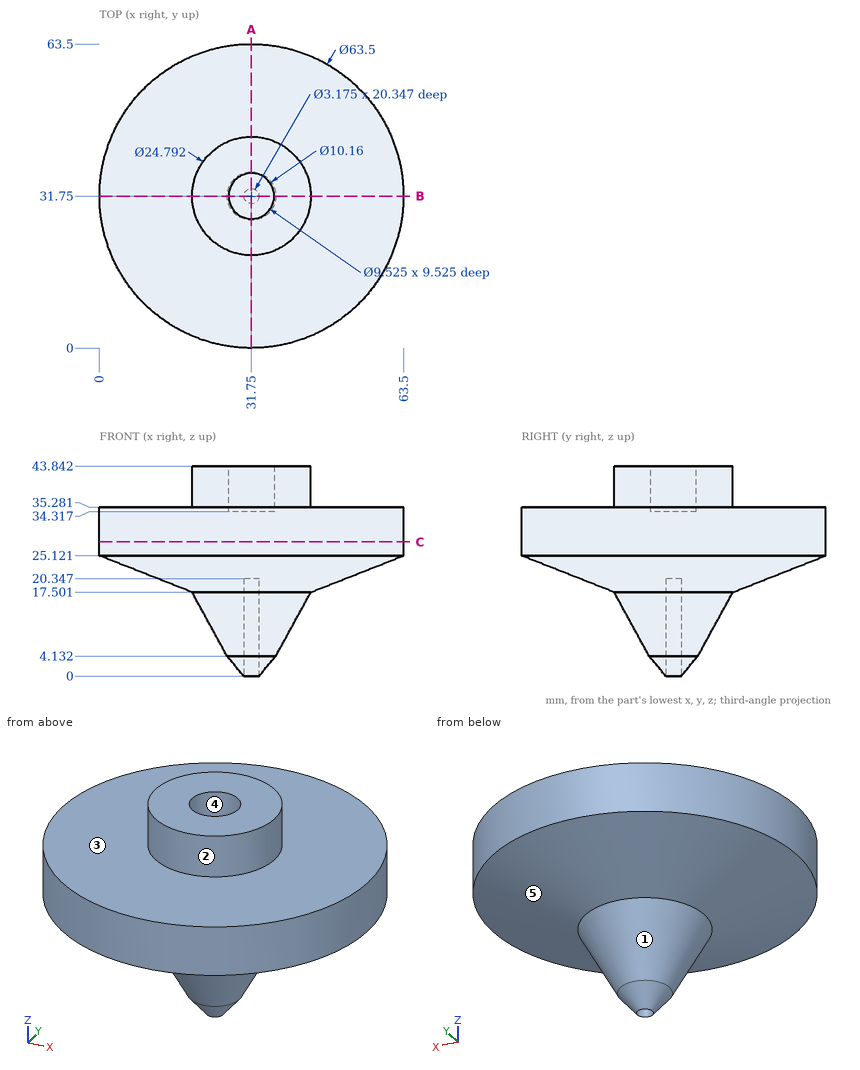
Check sheet for the drawn part. Datum: minimum x, y, z corner. Units: mm. A direction names the side the tool comes from. Round coordinates to 2 decimals unless told otherwise and drop trailing zeros. Write each loop counter-clockwise with the first axis right and the second up, starting at its lowest first coordinate (ties: lowest second). Pieces come first, ordered by that corner, then holes. Notation, with made-up numbers: (-15, 20) -> (21, 20) arc R26 cw to (21, 58) -> close; hole circle Ø3 at (-11.5, -16). An arc over 180 degrees is marked (long way). Put each result on its own line as item: value.
(1) Mould release check, pull along X, two halves, no side actions. Record for the marked faces 3, 4 and 5: released by +X, released by -X, zero draft, split by the parting line, or undercut.
Values found:
face 3: zero draft
face 4: undercut
face 5: split by the parting line
(2) Go/stop test with flat-tipped pins: pin 1 Ø4 at (x, y) = (40, 41) entering from -Z; pin 2 Ø8 at (y, z) = (49, 22.5) entering from -X; pin 3 Ø12 at (x, y) = (10, 13.5) entering from +Z. Record where each tip stops, or that it passes through.
Values found:
pin 1: stops at z = 13.84
pin 2: stops at x = 3.37
pin 3: stops at z = 35.28
(3) Material ranges on line 1 (Y direction, x = 31.75, z = 37.5); line 2 (X direction, y = 31, z = 12) (1 decimal); line 3 (Y direction, x = 31.75, z = 10.5) (1 decimal), recorded low to high.
Values found:
line 1: y = 19.35 to 26.99, 36.51 to 44.15
line 2: x = 22.4 to 30.4, 33.1 to 41.1
line 3: y = 23.2 to 30.2, 33.3 to 40.3
(4) Sectioned sample at A-A (x = 31.75). Enter the section's corners in (y, z).
Values found:
outline: (0, 25.12) -> (19.35, 17.5) -> (26.67, 4.13) -> (30.16, 0) -> (30.16, 20.35) -> (33.34, 20.35) -> (33.34, 0) -> (36.83, 4.13) -> (44.15, 17.5) -> (63.5, 25.12) -> (63.5, 35.28) -> (44.15, 35.28) -> (44.15, 43.84) -> (36.51, 43.84) -> (36.51, 34.32) -> (26.99, 34.32) -> (26.99, 43.84) -> (19.35, 43.84) -> (19.35, 35.28) -> (0, 35.28) -> close
(5) Sectioned sample at C-C (z = 28). Enter the section's corners in (x, y).
Values found:
outline: circle Ø63.5 at (31.75, 31.75)
(6) Tool access check on the marked faces 1 and 2. Record the directions out of +Z, -Z, +X, -X, +Y, -Y that give a thin tool (end or side, any length) a straight path to the whole face; none if there is none.
Values found:
face 1: -Z
face 2: +Z
